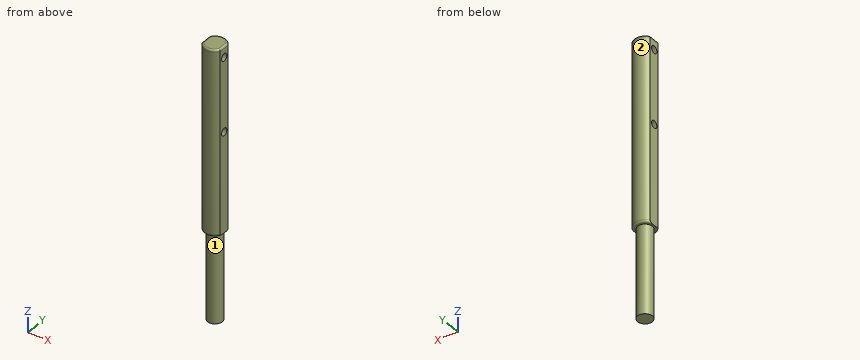
```python
from build123d import *

# Parameters (mm, degrees)
ESQUISSE1_R             = 20
BOSS_EXTRU_1_DEPTH      = 500
ESQUISSE1_4_R           = 20
BOSS_EXTRU_2_DEPTH      = 240
ESQUISSE2_R             = 10
ENL_V_MAT_EXTRU_1_DEPTH = 504.338852067
CONG_1_R                = 5


with BuildPart() as part:
    # Esquisse1 → Boss.-Extru.1 (new body)
    # profile 1 of 2: a face of its own
    with BuildSketch(Plane.XY):
        with BuildLine():
            ThreePointArc((25, 15), (0, 29.154759474), (-25, 15))
            Line((-25, 15), (-25, -15))
            ThreePointArc((-25, -15), (0, -29.154759474), (25, -15))
            Line((25, -15), (25, 15))
        make_face()
        Circle(ESQUISSE1_R, mode=Mode.SUBTRACT)
    # profile 2 of 2: a face of its own
    with BuildSketch(Plane.XY):
        Circle(ESQUISSE1_R)
    extrude(amount=BOSS_EXTRU_1_DEPTH)

    # Esquisse1<4> → Boss.-Extru.2 (add)
    with BuildSketch(Plane.XY):
        Circle(ESQUISSE1_4_R)
    extrude(amount=-BOSS_EXTRU_2_DEPTH)

    # Esquisse2 → Enlèv. mat.-Extru.1 (cut, through all)
    with BuildSketch(Plane.ZY.offset(25)):
        with Locations((470.845240526, 0)):
            Circle(ESQUISSE2_R)
        with Locations((270.845240526, 0)):
            Circle(ESQUISSE2_R)
    extrude(amount=-ENL_V_MAT_EXTRU_1_DEPTH, mode=Mode.SUBTRACT)

    # Congé1
    # the kernel refuses this fillet: 5 mm, written as the material it takes off along each edge
    with BuildSketch(Plane(origin=(0, 0, 500), x_dir=(0.8826697936069986, -0.46999365469522936, 0), z_dir=(-0.46999365469522936, -0.8826697936069986, 0))) as cong_1_piece_1:
        with BuildLine():
            CenterArc((29.154759474 - CONG_1_R, -CONG_1_R), CONG_1_R, 0, 90)
            Line((29.154759474, -CONG_1_R), (29.154759474 + CONG_1_R * 0.02, -CONG_1_R))
            Line((29.154759474 + CONG_1_R * 0.02, -CONG_1_R), (29.154759474 + CONG_1_R * 0.02, CONG_1_R * 0.02))
            Line((29.154759474 + CONG_1_R * 0.02, CONG_1_R * 0.02), (29.154759474 - CONG_1_R, CONG_1_R * 0.02))
            Line((29.154759474 - CONG_1_R, CONG_1_R * 0.02), (29.154759474 - CONG_1_R, 0))
        make_face()
    revolve(axis=Axis((0, 0, 500), (0, 0, 1)), revolution_arc=236.067769297, mode=Mode.SUBTRACT)
    with BuildSketch(Plane(origin=(0, 0, 500), x_dir=(-0.8826697936069986, 0.4699936546952294, 0), z_dir=(0.4699936546952294, 0.8826697936069986, 0))) as cong_1_piece_2:
        with BuildLine():
            CenterArc((29.154759474 - CONG_1_R, -CONG_1_R), CONG_1_R, 0, 90)
            Line((29.154759474 - CONG_1_R, 0), (29.154759474 - CONG_1_R, CONG_1_R * 0.02))
            Line((29.154759474 - CONG_1_R, CONG_1_R * 0.02), (29.154759474 + CONG_1_R * 0.02, CONG_1_R * 0.02))
            Line((29.154759474 + CONG_1_R * 0.02, CONG_1_R * 0.02), (29.154759474 + CONG_1_R * 0.02, -CONG_1_R))
            Line((29.154759474 + CONG_1_R * 0.02, -CONG_1_R), (29.154759474, -CONG_1_R))
        make_face()
    revolve(axis=Axis((0, 0, 500), (0, 0, 1)), revolution_arc=236.067769297, mode=Mode.SUBTRACT)
    with BuildSketch(Plane(origin=(-25, 45, 500), x_dir=(0, 0, -1), z_dir=(0, -1, 0)), Plane(origin=(25, -45, 500), x_dir=(0, 0, -1), z_dir=(0, 1, 0))) as cong_1_piece_3:
        with BuildLine():
            CenterArc((CONG_1_R, CONG_1_R), CONG_1_R, 180, 90)
            Line((0, CONG_1_R), (-CONG_1_R * 0.02, CONG_1_R))
            Line((-CONG_1_R * 0.02, CONG_1_R), (-CONG_1_R * 0.02, -CONG_1_R * 0.02))
            Line((-CONG_1_R * 0.02, -CONG_1_R * 0.02), (CONG_1_R, -CONG_1_R * 0.02))
            Line((CONG_1_R, -CONG_1_R * 0.02), (CONG_1_R, 0))
        make_face()
    extrude(amount=90, mode=Mode.SUBTRACT)
    with BuildSketch(Plane(origin=(0, 0, 0), x_dir=(-0.8826697936069986, 0.4699936546952294, 0), z_dir=(0.4699936546952294, 0.8826697936069986, 0))) as cong_1_piece_4:
        with BuildLine():
            CenterArc((29.154759474 - CONG_1_R, CONG_1_R), CONG_1_R, 270, 90)
            Line((29.154759474 - CONG_1_R, 0), (29.154759474 - CONG_1_R, -CONG_1_R * 0.02))
            Line((29.154759474 - CONG_1_R, -CONG_1_R * 0.02), (29.154759474 + CONG_1_R * 0.02, -CONG_1_R * 0.02))
            Line((29.154759474 + CONG_1_R * 0.02, -CONG_1_R * 0.02), (29.154759474 + CONG_1_R * 0.02, CONG_1_R))
            Line((29.154759474 + CONG_1_R * 0.02, CONG_1_R), (29.154759474, CONG_1_R))
        make_face()
    revolve(axis=Axis((0, 0, 0), (0, 0, 1)), revolution_arc=236.067769297, mode=Mode.SUBTRACT)
    with BuildSketch(Plane(origin=(0, 0, 0), x_dir=(0.8826697936069986, -0.46999365469522936, 0), z_dir=(-0.46999365469522936, -0.8826697936069986, 0))) as cong_1_piece_5:
        with BuildLine():
            CenterArc((29.154759474 - CONG_1_R, CONG_1_R), CONG_1_R, 270, 90)
            Line((29.154759474, CONG_1_R), (29.154759474 + CONG_1_R * 0.02, CONG_1_R))
            Line((29.154759474 + CONG_1_R * 0.02, CONG_1_R), (29.154759474 + CONG_1_R * 0.02, -CONG_1_R * 0.02))
            Line((29.154759474 + CONG_1_R * 0.02, -CONG_1_R * 0.02), (29.154759474 - CONG_1_R, -CONG_1_R * 0.02))
            Line((29.154759474 - CONG_1_R, -CONG_1_R * 0.02), (29.154759474 - CONG_1_R, 0))
        make_face()
    revolve(axis=Axis((0, 0, 0), (0, 0, 1)), revolution_arc=236.067769297, mode=Mode.SUBTRACT)


solid = part.part
```
Can you work these out from the model? Positions are in its coordinate system, mm. Face numbers are marked on the shaded views. A direction names the side the tool comes from. Coordinates: 2 decimals unless noted, no trailing zeros. Order: outer loops, then holes, each group sorted by start corner. A loop starts at its lowest first (then second) coordinate and runs counter-clockwise, first axis right, second up.
1. For the marked faces 1 and 2, which set-ups out of +Z, -Z, +X, -X, +Y, -Y let a thin tool reach every point of the face, with its end or its side?
2. I'm going to push flat-ended pins straight in: pin 1 (3 mm diameter, centred on y = 9, z = -65, fed in from +X); pin 2 (12 mm diameter, centred on y = 0, z = 470.85, fed in from +X); pin 3 (10 mm diameter, centred on x = 10.5, z = 385, fed in from -Y); pin 4 (3 mm diameter, centred on y = 18, z = 231.5, fed in from -X). Where does each tip first touch, or does it pass through?
3. If we section it at D-D (z = 197.5): Please give me the cut outline in (x, y).
4. I need wall thicknesses on line 1 (Z direction, x = -10, y = -2); line 2 (X direction, y = -0.5, z = -157.5); line 3 (Y direction, x = 2, z = 129). Which ranges of each line are inside material? Lowest first, please.
5. If we section it at A-A (y = 0): Please give me the cut outline in (x, z), then the cut area to 3 significant figures.
6. If we section it at B-B (x = 0): Please give me the cut outline in (y, z).
7. If we section it at C-C (z = -144): Please give me the cut outline in (x, y), then the cut area to 3 significant figures.
Entries:
1. face 1: -Z
1. face 2: +Z, -Z, +Y
2. pin 1: stops at x = 18.54
2. pin 2: passes through
2. pin 3: stops at y = -28.63
2. pin 4: stops at x = -24.04
3. outline: (-25, -15) arc R29.15 ccw to (25, -15) - (25, 15) arc R29.15 ccw to (-25, 15) - close
4. line 1: z = -240 to 261.05, 280.64 to 461.05, 480.64 to 500
4. line 2: x = -19.99 to 19.99
4. line 3: y = -29.09 to 29.09
5. outline: (-25, 0.07) arc R5 ccw to (-24.15, 0) - (-20, 0) - (-20, -240) - (20, -240) - (20, 0) - (24.15, 0) arc R5 ccw to (25, 0.07) - (25, 260.85) - (-25, 260.85) - close; (-25, 280.85) - (25, 280.85) - (25, 460.85) - (-25, 460.85) - close; (-25, 480.85) - (25, 480.85) - (25, 495) arc R5 ccw to (20, 500) - (-20, 500) arc R5 ccw to (-25, 495) - close
5. area: 32,600 mm2
6. outline: (-29.15, 5) arc R5 ccw to (-24.15, 0) - (-20, 0) - (-20, -240) - (20, -240) - (20, 0) - (24.15, 0) arc R5 ccw to (29.15, 5) - (29.15, 495) arc R5 ccw to (24.15, 500) - (-24.15, 500) arc R5 ccw to (-29.15, 495) - close; hole circle Ø20 at (0, 270.85); hole circle Ø20 at (0, 470.85)
7. outline: circle Ø40 at (0, 0)
7. area: 1,260 mm2
